from build123d import *

# Parameters (mm, degrees)
F1_DEPTH  = 10
F2_W      = 37
F2_H      = 36
F3_DEPTH  = 10
F4_R      = 1.25
F5_DEPTH  = 25
F6_W      = 27
F6_H      = 25
F7_DEPTH  = 8
F8_R      = 1.25
F9_DEPTH  = 36.001
F10_R     = 1.25
F11_DEPTH = 42.001
F13_R     = 15
F14_DEPTH = 10
F15_DEPTH = 10
F16_R     = 6.5
F17_DEPTH = 10.001


with BuildPart() as f1:
    # F0 (on Front) → F1 (new body)
    with BuildSketch(Plane.XZ):
        with BuildLine():
            Line((-18.5, -18), (18.5, -18))
            ThreePointArc((18.5, -18), (20.267767, -17.267767), (21, -15.5))
            Line((21, -15.5), (21, 15.5))
            ThreePointArc((21, 15.5), (20.267767, 17.267767), (18.5, 18))
            Line((18.5, 18), (-18.5, 18))
            ThreePointArc((-18.5, 18), (-20.267767, 17.267767), (-21, 15.5))
            Line((-21, 15.5), (-21, -15.5))
            ThreePointArc((-21, -15.5), (-20.267767, -17.267767), (-18.5, -18))
        make_face()
    extrude(amount=-F1_DEPTH)

    # F2 (on face) → F3 (join)
    with BuildSketch(Plane.XZ):
        Rectangle(F2_W, F2_H)
    extrude(amount=F3_DEPTH)

    # F4 (on face) → F5 (cut)
    with BuildSketch(Plane(origin=(0, 10, 0), x_dir=(-1, 0, 0), z_dir=(0, 1, 0))):
        with Locations((-17.5, 14.5)):
            Circle(F4_R)
        with Locations((17.5, 14.5)):
            Circle(F4_R)
        with Locations((-17.5, -14.5)):
            Circle(F4_R)
        with Locations((17.5, -14.5)):
            Circle(F4_R)
    extrude(amount=-F5_DEPTH, mode=Mode.SUBTRACT)

    # F6 (on face) → F7 (cut)
    with BuildSketch(Plane(origin=(0, 10, 0), x_dir=(-1, 0, 0), z_dir=(0, 1, 0))):
        Rectangle(F6_W, F6_H)
    extrude(amount=-F7_DEPTH, mode=Mode.SUBTRACT)

    # F8 (on face) → F9 (cut, through all)
    with BuildSketch(Plane.XY.offset(18)):
        with Locations((0, 5)):
            Circle(F8_R)
        with Locations((0, -5)):
            Circle(F8_R)
    extrude(amount=-F9_DEPTH, mode=Mode.SUBTRACT)

    # F10 (on face) → F11 (cut, through all)
    with BuildSketch(Plane.YZ.offset(21)):
        with Locations((5, 0)):
            Circle(F10_R)
        with Locations((-5, 0)):
            Circle(F10_R)
    extrude(amount=-F11_DEPTH, mode=Mode.SUBTRACT)

    # F13 (on face) → F14 (cut)
    with BuildSketch(Plane.XZ.offset(10)):
        Circle(F13_R)
    extrude(amount=-F14_DEPTH, mode=Mode.SUBTRACT)

    # F12 (on face) → F15 (cut)
    with BuildSketch(Plane.XZ.offset(10)):
        with BuildLine():
            ThreePointArc((0, -18), (-18, 0), (0, 18))
            Line((0, 18), (-18.5, 18))
            Line((-18.5, 18), (-18.5, 15.25))
            ThreePointArc((-18.5, 15.25), (-16.25, 14.5), (-18.5, 13.75))
            Line((-18.5, 13.75), (-18.5, -13.75))
            ThreePointArc((-18.5, -13.75), (-16.25, -14.5), (-18.5, -15.25))
            Line((-18.5, -15.25), (-18.5, -18))
            Line((-18.5, -18), (0, -18))
        make_face()
        with BuildLine():
            ThreePointArc((0, 18), (12.727922, 12.727922), (18, 0))
            ThreePointArc((18, 0), (12.727922, -12.727922), (0, -18))
            Line((0, -18), (18.5, -18))
            Line((18.5, -18), (18.5, -15.25))
            ThreePointArc((18.5, -15.25), (17.104715, -15.685854), (16.25, -14.5))
            ThreePointArc((16.25, -14.5), (17.104715, -13.314146), (18.5, -13.75))
            Line((18.5, -13.75), (18.5, 13.75))
            ThreePointArc((18.5, 13.75), (17.104715, 13.314146), (16.25, 14.5))
            ThreePointArc((16.25, 14.5), (17.104715, 15.685854), (18.5, 15.25))
            Line((18.5, 15.25), (18.5, 18))
            Line((18.5, 18), (0, 18))
        make_face()
    extrude(amount=-F15_DEPTH, mode=Mode.SUBTRACT)

    # F16 (on face) → F17 (cut, through all)
    with BuildSketch(Plane.XZ):
        Circle(F16_R)
    extrude(amount=-F17_DEPTH, mode=Mode.SUBTRACT)


solid = f1.part
Design review of the part built by this model. Coordinates are the model's own, in mm. A direction names the side the tool comes from. Give positions to 0.01 mm unless a question says otherwise; leave off trailing zeros. Order: outer loops, then holes, each group sorted by start corner. A loop starts at its lowest first (then second) coordinate and runs counter-clockwise, first axis right, second up.
1. Add section D-D, the plane y = -5. State the section outline as (x, z) points.
Solution:
outline: (-17.96, -1.25) arc R18 ccw to (-1.25, -17.96) - (-1.25, -14.95) arc R15 cw to (-14.95, -1.25) - close; (-17.96, 1.25) - (-14.95, 1.25) arc R15 cw to (-1.25, 14.95) - (-1.25, 17.96) arc R18 ccw to start; (1.25, -17.96) arc R18 ccw to (17.96, -1.25) - (14.95, -1.25) arc R15 cw to (1.25, -14.95) - close; (1.25, 14.95) arc R15 cw to (14.95, 1.25) - (17.96, 1.25) arc R18 ccw to (1.25, 17.96) - close
2. Add section C-C, the plane z = -4. State the section outline as (x, y) points, then the cut area to 3 significant figures.
Solution:
outline: (-21, 0) - (-17.55, 0) - (-17.55, -10) - (-14.46, -10) - (-14.46, 0) - (-5.12, 0) - (-5.12, 2) - (-13.5, 2) - (-13.5, 10) - (-21, 10) - close; (5.12, 0) - (14.46, 0) - (14.46, -10) - (17.55, -10) - (17.55, 0) - (21, 0) - (21, 10) - (13.5, 10) - (13.5, 2) - (5.12, 2) - close
area: 245 mm2
3. Add section A-A, the plane y = 5. State how many separate pieces and enclosed holes the cut face has, then the cut area to 3 significant figures.
Solution:
separate pieces: 4
enclosed holes: 4
area: 747 mm2
4. To check wall thickness, follow L1, parallel to Z at x = -18.25, y = 5; L2, parallel to Z at x = 17.5, y = 2.5; L3, parallel to X at y = 5.75, z = -2.5. State the ranges of each line that lie inside material, in increasing order.
Solution:
L1: z = -18 to -15.5, -13.5 to -1.25, 1.25 to 13.5, 15.5 to 18
L2: z = -18 to -15.75, -13.25 to 13.25, 15.75 to 18
L3: x = -21 to -13.5, 13.5 to 21
5. Add section B-B, the plane x = -17.5. State the section outline as (y, z) points.
Solution:
outline: (-10, -4.21) - (0, -4.21) - (0, -13.25) - (10, -13.25) - (10, 13.25) - (0, 13.25) - (0, 4.21) - (-10, 4.21) - close; (0, -18) - (10, -18) - (10, -15.75) - (0, -15.75) - close; (0, 15.75) - (10, 15.75) - (10, 18) - (0, 18) - close; hole circle Ø2.5 at (-5, 0); hole circle Ø2.5 at (5, 0)
6. For pin 1 Ø6 at (y, z) = (-6, -0.5) entering from -X; pin 2 Ø6.5 at (x, z) = (-9.5, -4.5) entering from -Y, all flat-tipped, find the tip position at first contact; note any pin that passes through.
Solution:
pin 1: stops at x = -18
pin 2: stops at y = 0
7. Mouldability with a two-part tool opening along Y and no side actions: class faces 1 (the flat face through (3, 2, 6)), 2 (the cylindrical face through (17.3, 3.75, 0.05)), 3 (the flat face through (-13.5, 7, 0)) as +Y half, -Y half, draft (parallel to the pull), parting line (faces both ways), or undercut.
Solution:
face 1: +Y half
face 2: undercut
face 3: draft
8. Tool access review of faces 4 (the cylindrical face through (13.856, -5.07, -5.745)), 5 (the cylindrical face through (-16.45, -6.25, 0.05)), 6 (the flat face through (18.2, 0, 0.1)), 7 (the flat face through (13.5, 7, 0)), 8 (the flat face through (-18.3, 0, 1.4)): name each direction out of +Z, -Z, +X, -X, +Y, -Y from which nothing blocks a thin tool from reaching the whole face with its end or side.
Solution:
face 4: -Y
face 5: +X, -X
face 6: +X, -Y
face 7: +Y
face 8: -X, -Y
